Print and shaded views of the part. All mm, measured from the part's lowest x, y and z. Give positions to 0.01 mm unless a question says otherwise; leave off trailing zeros. Write each loop counter-clockwise with the first axis right and the second up, starting at its lowest first coordinate (ties: lowest second). Pieces come first, ordered by that corner, then holes. Notation, with made-up numbers: (73.5, 8) -> (80.5, 8) arc R26 cw to (80.5, 36) -> close; hole circle Ø10 at (8, -33.5). An arc over 180 degrees is marked (long way). Put each result on its own line as item: value.
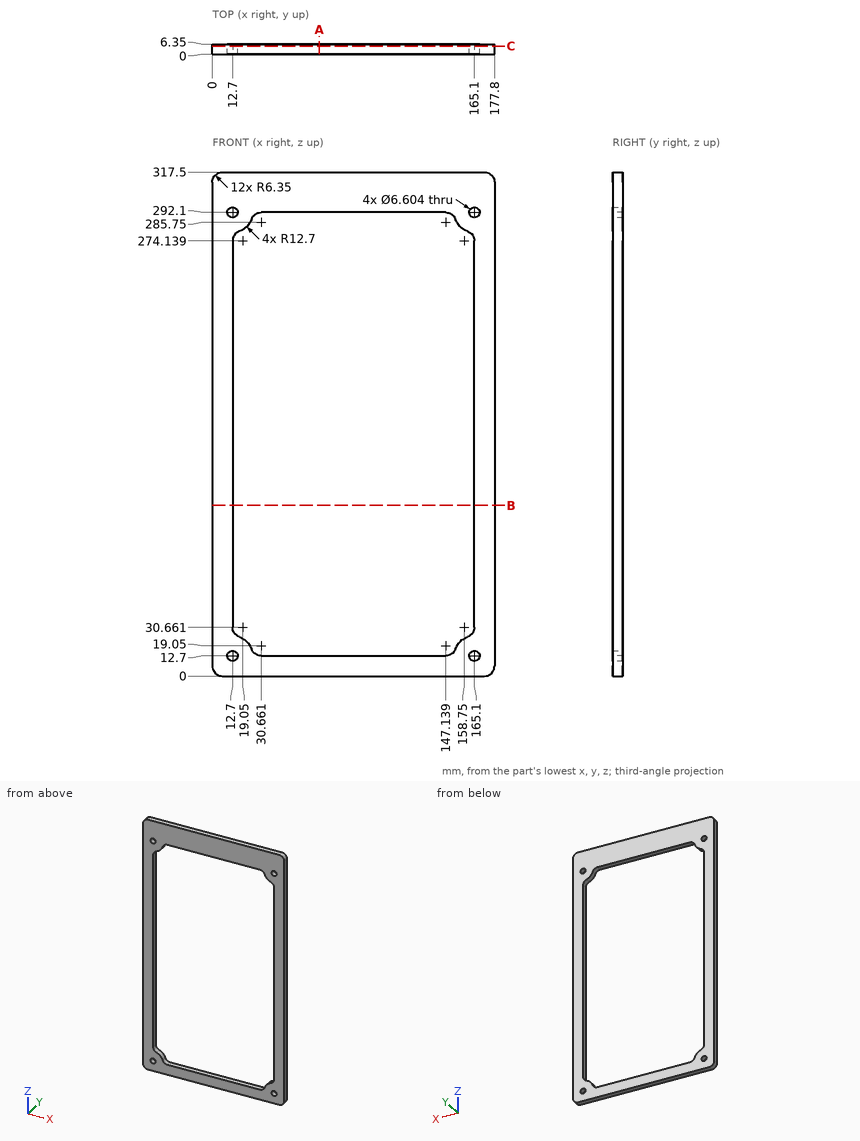
1) Slice it at B-B (z = 107.5). Write the cut outline in (x, y), plus the area to 3 significant figures.
Filled sheet:
outline: (0, 0) -> (12.7, 0) -> (12.7, 6.35) -> (0, 6.35) -> close; (165.1, 0) -> (177.8, 0) -> (177.8, 6.35) -> (165.1, 6.35) -> close
area: 161 mm2
2) Pin check, flat tips, straight feed: pin 1 (1 mm diameter, centred on x = 118.5, y = 5.5, fed in from -Z); pin 2 (4 mm diameter, centred on x = 165.1, z = 292.1, fed in from -Y). Stop position of each tip, or through.
Filled sheet:
pin 1: z = 0
pin 2: through
3) Wall check: L1, parallel to X at y = 3.5, z = 93.5; L2, parallel to Z at x = 60, y = 1.75; L3, parallel to Z at x = 168, y = 1 (1 decimal). Give the ranges that are in metal, low to high.
Filled sheet:
L1: 0 to 12.7, 165.1 to 177.8
L2: 0 to 12.7, 292.1 to 317.5
L3: 0 to 11.1, 14.3 to 290.5, 293.7 to 317.5
4) Slice it at A-A (x = 67.5). Write the cut outline in (y, z).
Filled sheet:
outline: (0, 0) -> (6.35, 0) -> (6.35, 12.7) -> (0, 12.7) -> close; (0, 292.1) -> (6.35, 292.1) -> (6.35, 317.5) -> (0, 317.5) -> close
5) Slice it at C-C (y = 5). Write the cut outline in (x, z), plus the area to 3 significant figures.
Filled sheet:
outline: (0, 6.35) arc R6.35 ccw to (6.35, 0) -> (171.45, 0) arc R6.35 ccw to (177.8, 6.35) -> (177.8, 311.15) arc R6.35 ccw to (171.45, 317.5) -> (6.35, 317.5) arc R6.35 ccw to (0, 311.15) -> close; hole circle Ø6.6 at (12.7, 12.7); hole circle Ø6.6 at (12.7, 292.1); hole (12.7, 30.66) arc R6.35 ccw to (16.93, 24.67) arc R12.7 cw to (24.67, 16.93) arc R6.35 ccw to (30.66, 12.7) -> (147.14, 12.7) arc R6.35 ccw to (153.13, 16.93) arc R12.7 cw to (160.87, 24.67) arc R6.35 ccw to (165.1, 30.66) -> (165.1, 274.14) arc R6.35 ccw to (160.87, 280.13) arc R12.7 cw to (153.13, 287.87) arc R6.35 ccw to (147.14, 292.1) -> (30.66, 292.1) arc R6.35 ccw to (24.67, 287.87) arc R12.7 cw to (16.93, 280.13) arc R6.35 ccw to (12.7, 274.14) -> close; hole circle Ø6.6 at (165.1, 12.7); hole circle Ø6.6 at (165.1, 292.1)
area: 14,200 mm2
